Source: three-view drawing plus pictorial views. Frame: mm from the lowest corner of the part. Give positions to 0.01 mm unless a question says otherwise; leave off trailing zeros. Loops run counter-clockwise (first coordinate to the right, second up) from the corner with the lowest first, then second, coordinate; pieces in that order, holes last. Notation, with made-up numbers: (-31.75, 55) - (23.25, 55) arc R16 cw to (23.25, 76) - close; hole circle Ø3 at (3.5, 40.5). An arc over 180 degrees is marked (long way). Write each question's results on one line, items separated by ' | '. Start each with the question number.
(1) Contact query for a flat-ended pin moving along its axis: pin 1 (1.5 mm diameter, centred on x = 23, y = 13.5, fed in from -Z). Output: stop coordinate, or through.
(2) Cut plane B-B on x = 5.43. Return the cut outline in (y, z).
(3) Cut plane C-C on y = 20. Return the cut outline in (x, z).
(4) Material intervals for line 1 along Z through (x, y) = (52.57, 16); line 2 along X through (y, z) = (47, 6.5); line 3 along X through (y, z) = (14.5, 6), sorted ascending. Write a range as [from, to].
(5) Cut plane A-A on z = 4.76. Return the cut outline in (x, y).
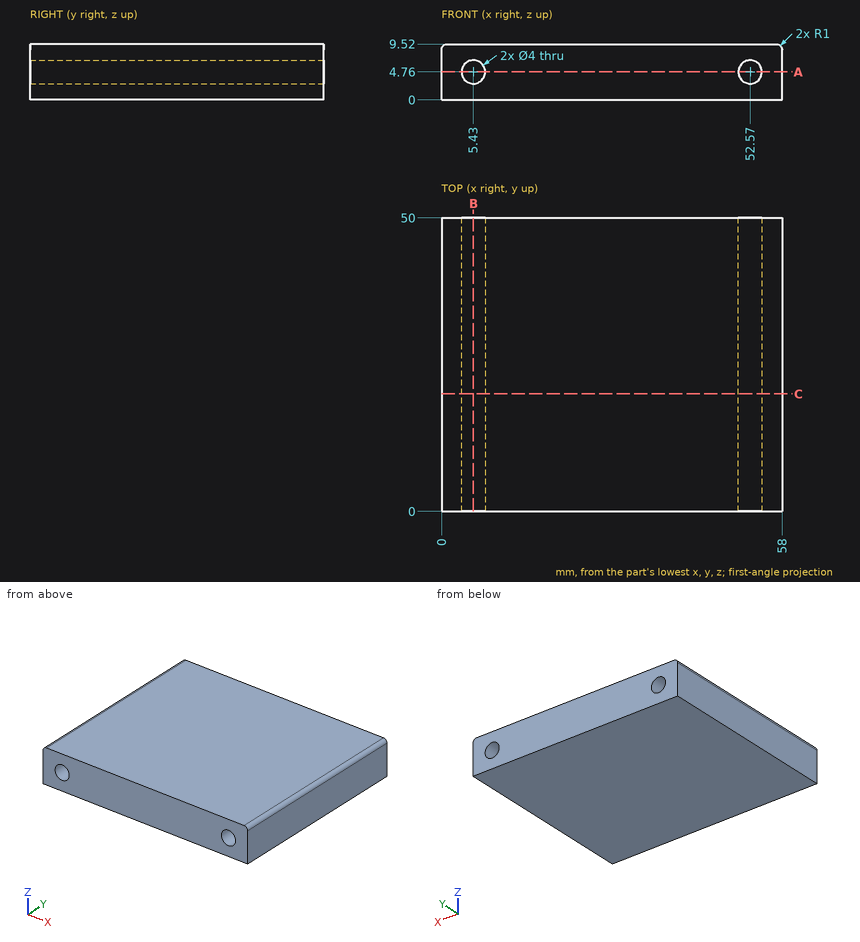
Ans:
1) pin 1: z = 0
2) outline: (0, 0) - (50, 0) - (50, 2.76) - (0, 2.76) - close; (0, 6.76) - (50, 6.76) - (50, 9.52) - (0, 9.52) - close
3) outline: (0, 0) - (58, 0) - (58, 8.52) arc R1 ccw to (57, 9.52) - (1, 9.52) arc R1 ccw to (0, 8.52) - close; hole circle Ø4 at (5.43, 4.76); hole circle Ø4 at (52.57, 4.76)
4) line 1: [0, 2.76], [6.76, 9.52] | line 2: [0, 4.44], [6.42, 51.58], [53.56, 58] | line 3: [0, 3.86], [7, 51], [54.14, 58]
5) outline: (0, 0) - (3.43, 0) - (3.43, 50) - (0, 50) - close; (7.43, 0) - (50.57, 0) - (50.57, 50) - (7.43, 50) - close; (54.57, 0) - (58, 0) - (58, 50) - (54.57, 50) - close
